CAD build for the part. Positions are in the model's coordinates, mm. A direction names the side the tool comes from. Coordinates: 2 decimals unless noted, no trailing zeros. Write each loop counter-clockwise with the first axis right and the second up, starting at its lowest first coordinate (ties: lowest second). Pieces come first, ordered by that corner, then holes. Notation, with made-up numbers: (7, 41.5) - (18, 41.5) arc R9 ccw to (18, 56.5) - close; hole circle Ø9 at (72, 58.5). An arc over 180 degrees is marked (long way). Answer in a Markdown table with one row per item. Add a question column.
Q1. Band-saw the part on C-C (y = 42). List the corners of the cut face in (x, z), and give its area (3 significant figures).
Q2. Pin check, flat tip, straight feed: pin 1 (1 mm diameter, centred on x = 12, y = 41, fed in from -Z). Stop position of the tip, or through.
Q3. Band-saw the part on D-D (x = -25). List the corners of the cut face in (y, z).
Q4. Band-saw the part on A-A (x = 6.5). List the corners of the cut face in (y, z), and give its area (3 significant figures).
Q5. Band-saw the part on B-B (z = -2). List the corners of the cut face in (x, y), and give its area (3 significant figures).
Q6. 3-axis set-ups, long thin cutter, end or side, ignore diameter. For faces 1 (the flat face through (0, 20, 30)), 2 (the flat face through (0, 40, -20)): which of +Z, -Z, +X, -X, +Y, -Y reach the whole face in a straight line?
Q7. Drill centre lines: line 1 along Y through (x, z) = (-19, -17.5); line 2 along X through (y, z) = (50.5, 10); line 3 along X through (y, z) = (57, -1.5). Where is each one in solid material? Low to high. Write a range as from..to.
```python
from build123d import *

# Parameters (mm, degrees)
SKETCH1_W           = 60
SKETCH1_H           = 60
BOSS_EXTRUDE1_DEPTH = 40
SKETCH2_W           = 30
SKETCH2_H           = 30
BOSS_EXTRUDE2_DEPTH = 20
BOSS_EXTRUDE2_TAPER = 5
DRAFT1_START        = -16
DRAFT1_DEPTH        = 32
DRAFT1_2_DEPTH      = 32


with BuildPart() as part:
    # Sketch1 → Boss-Extrude1 (new body)
    with BuildSketch(Plane(origin=(0, 0, 0), x_dir=(1, 0, 0), z_dir=(0, 1, 0))):
        Rectangle(SKETCH1_W, SKETCH1_H)
    extrude(amount=BOSS_EXTRUDE1_DEPTH)

    # Sketch2 → Boss-Extrude2 (add)
    with BuildSketch(Plane(origin=(0, 40, 0), x_dir=(1, 0, 0), z_dir=(0, 1, 0))):
        Rectangle(SKETCH2_W, SKETCH2_H)
    extrude(amount=BOSS_EXTRUDE2_DEPTH, taper=BOSS_EXTRUDE2_TAPER)

    # Draft1: read off the stored shape, not the designer's step
    # Draft1 outline → Draft1 (cut)
    with BuildSketch(Plane.XY.offset(DRAFT1_START)):
        Polygon((-15, 40), (-12.544308782, 60), (-13.250226729, 60), align=None)
        Polygon((12.544308782, 60), (15, 40), (13.250226729, 60), align=None)
    extrude(amount=DRAFT1_DEPTH, mode=Mode.SUBTRACT)

    # Draft1 2 outline → Draft1 2 (cut)
    with BuildSketch(Plane.YZ.offset(DRAFT1_START)):
        Polygon((60, -12.544308782), (40, -15), (60, -13.250226729), align=None)
        Polygon((60, 13.250226729), (40, 15), (60, 12.544308782), align=None)
    extrude(amount=DRAFT1_2_DEPTH, mode=Mode.SUBTRACT)


solid = part.part
```
Checked values:
| question | item | result |
|---|---|---|
| 1 | outline | (-14.75, -14.75) - (14.75, -14.75) - (14.75, 14.75) - (-14.75, 14.75) - close |
| 1 | area | 871 mm² |
| 2 | pin 1 | stops at z = -14.94 |
| 3 | outline | (0, -30) - (40, -30) - (40, 30) - (0, 30) - close |
| 4 | outline | (0, -30) - (40, -30) - (40, -15) - (60, -12.54) - (60, 12.54) - (40, 15) - (40, 30) - (0, 30) - close |
| 4 | area | 2,950 mm² |
| 5 | outline | (-30, 0) - (30, 0) - (30, 40) - (15, 40) - (12.54, 60) - (-12.54, 60) - (-15, 40) - (-30, 40) - close |
| 5 | area | 2,950 mm² |
| 6 | face 1 | +Z, +X, -X, +Y, -Y |
| 6 | face 2 | +Y |
| 7 | line 1 | y = 0..40 |
| 7 | line 2 | x = -13.71..13.71 |
| 7 | line 3 | x = -12.91..12.91 |
